Design review of the part shown in the three views and the two pictorial views. Dimensions are in mm from the part's minimum x, y and z. A direction names the side the tool comes from. Round coordinates to 2 decimals unless told otherwise and drop trailing zeros. Write each loop counter-clockwise with the first axis right and the second up, starting at its lowest first coordinate (ties: lowest second). Pieces come first, ordered by that corner, then holes. Notation, with made-up numbers: (25, -16) - (47, -16) arc R13 ccw to (47, -11) - close; hole circle Ø2 at (43, -28). An arc over 180 degrees is marked (long way). One line per item, written item: value. Start each with the question number.
Q1. For probe 1 along X at (y, z) = (4, 46); probe 2 along X at (y, z) = (7.5, 20); probe 3 along Z at (x, y) = (83, 20.55), list the stretches that pass through material, from the lowest coordinate up.
Q2. Add section C-C on z = 20. Write out the cut boundary in (x, y), and give its area (3 significant figures).
Q3. Add section A-A on y = 12.5. Write out the cut boundary in (x, z), and give its area (3 significant figures).
Q4. Tool access review of the marked faces 1, 2 and 3: name each direction out of +Z, -Z, +X, -X, +Y, -Y from which nothing blocks a thin tool from reaching the whole face with its end or side.
Q5. Add section D-D on x = 28. Write out the cut boundary in (y, z).
Q6. Add section B-B on x = 13.5. Write out the cut boundary in (y, z), and give its area (3 significant figures).
Q7. Mouldability with a two-part tool opening along X and no side actions: class the marked faces 4, 5 and 6 as +X half, -X half, draft (parallel to the pull), parting line (faces both ways), or undercut.
Q8. Clearance check with flat-ended pins moving along their axes: pin 1 Ø8 at (x, y) = (72.5, 22.5) entering from -Z; pin 2 Ø3 at (x, z) = (27, 20.5) entering from -Y; pin 3 Ø4 at (x, z) = (26.5, 18) entering from +Y; pin 4 Ø1.5 at (x, y) = (25, 18) entering from +Z. State where each tip first meets the part, or that it passes through.
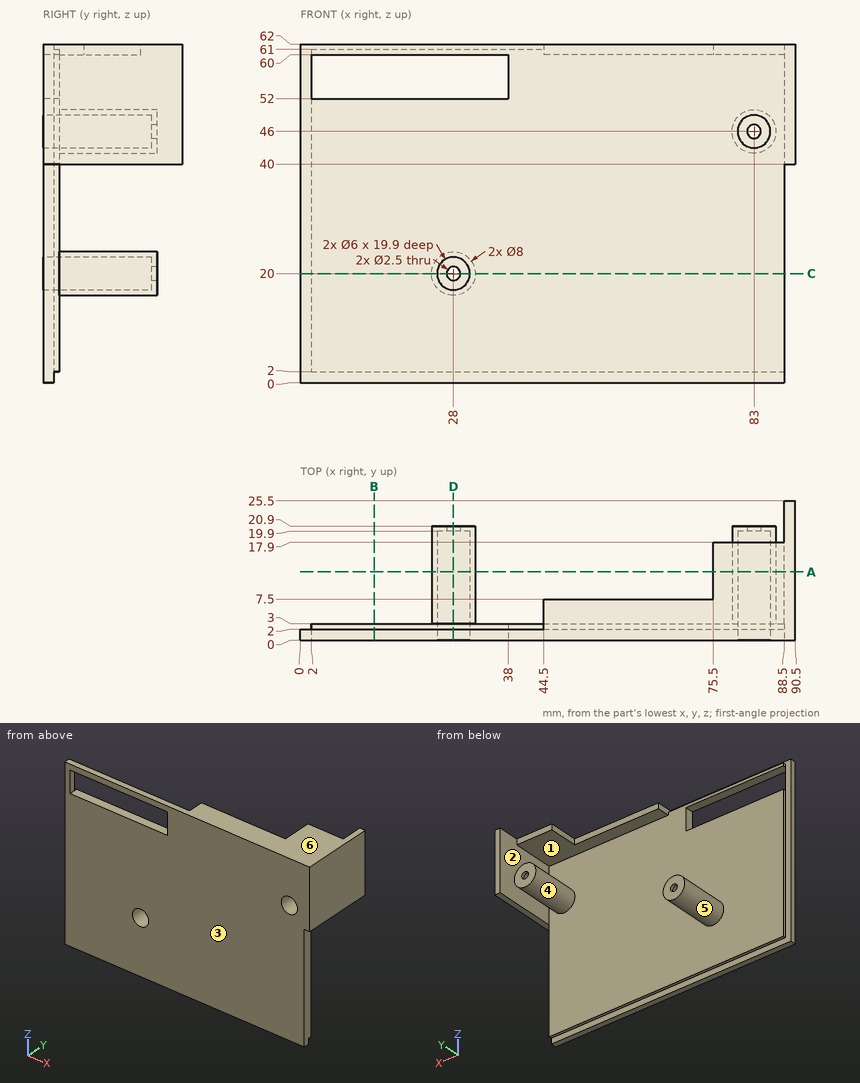
Result set:
1. probe 1: x = 79 to 80, 86 to 87, 88.5 to 90.5
1. probe 2: x = 24 to 25, 31 to 32
1. probe 3: z = 42 to 44.75, 47.25 to 50
2. outline: (0, 0) - (25, 0) - (25, 19.9) - (26.75, 19.9) - (26.75, 20.9) - (24, 20.9) - (24, 3) - (2, 3) - (2, 2) - (0, 2) - close; (29.25, 19.9) - (31, 19.9) - (31, 0) - (88.5, 0) - (88.5, 3) - (32, 3) - (32, 20.9) - (29.25, 20.9) - close
2. area: 285 mm^2
3. outline: circle Ø8 at (28, 20); (75.5, 60) - (88.5, 60) - (88.5, 40) - (90.5, 40) - (90.5, 62) - (75.5, 62) - close; circle Ø8 at (83, 46); hole circle Ø6 at (28, 20); hole circle Ø6 at (83, 46)
3. area: 114 mm^2
4. face 1: -X, +Y
4. face 2: -Z, +Y
4. face 3: +Z, -Z, +X, -X, -Y
5. outline: (0, 0) - (2, 0) - (2, 2) - (3, 2) - (3, 16) - (20.9, 16) - (20.9, 18.75) - (19.9, 18.75) - (19.9, 17) - (0, 17) - close; (0, 23) - (19.9, 23) - (19.9, 21.25) - (20.9, 21.25) - (20.9, 24) - (3, 24) - (3, 52) - (0, 52) - close; (0, 60) - (3, 60) - (3, 61) - (2, 61) - (2, 62) - (0, 62) - close
6. outline: (0, 0) - (2, 0) - (2, 2) - (3, 2) - (3, 52) - (0, 52) - close; (0, 60) - (3, 60) - (3, 61) - (2, 61) - (2, 62) - (0, 62) - close
6. area: 159 mm^2
7. face 4: undercut
7. face 5: parting line
7. face 6: draft
8. pin 1: passes through
8. pin 2: stops at y = 19.9
8. pin 3: stops at y = 20.9
8. pin 4: stops at z = 23.31
